Design review of the part built by this model. Coordinates are the model's own, in mm. Coordinates: 2 decimals unless noted, no trailing zeros. Write each loop counter-clockwise with the first axis right and the second up, starting at its lowest first coordinate (ties: lowest second). Pieces come first, ordered by that corner, then holes. Notation, with made-up numbers: M 86,12 L 120,12 A27 ccw 120,42 Z; hole C 40.5,28 d8. An arc over 180 degrees is marked long. One line per question, with ' | ' between items.
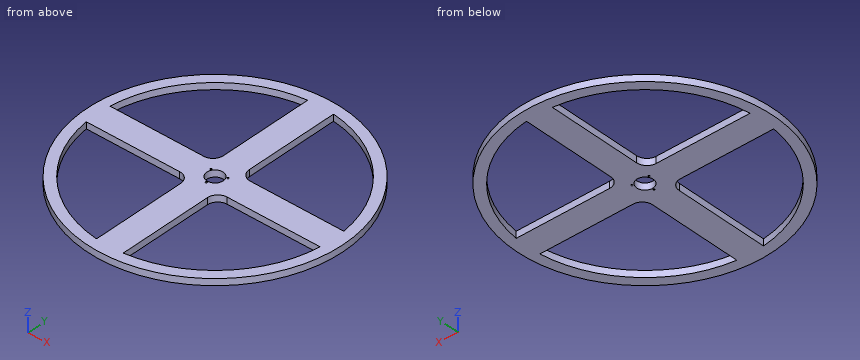
from build123d import *

# Parameters (mm, degrees)
SKETCH1_R           = 123.5325
SKETCH1_R_2         = 113.71
BOSS_EXTRUDE1_DEPTH = 6.35
CUT_EXTRUDE1_REACH  = 176.817
SKETCH2_R           = 7.937515
CUT_EXTRUDE2_REACH  = 176.817
SKETCH3_R           = 0.79375


with BuildPart() as part:
    # Sketch1 → Boss-Extrude1 (new body)
    # profile 1 of 2: a face of its own
    with BuildSketch(Plane.XY):
        Circle(SKETCH1_R)
        Circle(SKETCH1_R_2, mode=Mode.SUBTRACT)
    # profile 2 of 2: a face of its own
    with BuildSketch(Plane.XY):
        with BuildLine():
            ThreePointArc((22.7, 12.7), (15.628932188, 15.628932188), (12.7, 22.7))
            Line((12.7, 22.7), (12.7, 112.998557955))
            ThreePointArc((12.7, 112.998557955), (0.173278497, 113.709867974), (-12.355552704, 113.036739237))
            Line((-12.355552704, 113.036739237), (-12.355552704, 22.7))
            ThreePointArc((-12.355552704, 22.7), (-15.284484892, 15.628932188), (-22.355552704, 12.7))
            Line((-22.355552704, 12.7), (-112.998557955, 12.7))
            ThreePointArc((-112.998557955, 12.7), (-113.71, 0), (-112.998557955, -12.7))
            Line((-112.998557955, -12.7), (-22.7, -12.7))
            ThreePointArc((-22.7, -12.7), (-15.628932188, -15.628932188), (-12.7, -22.7))
            Line((-12.7, -22.7), (-12.7, -112.998557955))
            ThreePointArc((-12.7, -112.998557955), (0.173337872, -113.709867883), (13.044447296, -112.959313448))
            Line((13.044447296, -112.959313448), (13.044447296, -22.7))
            ThreePointArc((13.044447296, -22.7), (15.973379485, -15.628932188), (23.044447296, -12.7))
            Line((23.044447296, -12.7), (112.998557955, -12.7))
            ThreePointArc((112.998557955, -12.7), (113.53200017, -6.359955774), (113.71, 0))
            ThreePointArc((113.71, 0), (113.53200017, 6.359955774), (112.998557955, 12.7))
            Line((112.998557955, 12.7), (22.7, 12.7))
        make_face()
    extrude(amount=BOSS_EXTRUDE1_DEPTH)

    # Sketch2 → Cut-Extrude1 (cut, up to next)
    with BuildSketch(Plane.XY.offset(6.35), mode=Mode.PRIVATE) as cut_extrude1_sk1:
        Circle(SKETCH2_R)
    cut_extrude1_tool1 = extrude(cut_extrude1_sk1.sketch, amount=-CUT_EXTRUDE1_REACH, mode=Mode.PRIVATE) & part.part
    add(cut_extrude1_tool1.solids().sort_by_distance((0, 0, 6.35))[0], mode=Mode.SUBTRACT)

    # Sketch3 → Cut-Extrude2 (cut, up to next)
    with BuildSketch(Plane.XY.offset(6.35), mode=Mode.PRIVATE) as cut_extrude2_sk1:
        with Locations((0, -9.525)):
            Circle(SKETCH3_R)
    cut_extrude2_tool1 = extrude(cut_extrude2_sk1.sketch, amount=-CUT_EXTRUDE2_REACH, mode=Mode.PRIVATE) & part.part
    # Sketch3 → Cut-Extrude2 (cut, up to next)
    with BuildSketch(Plane.XY.offset(6.35), mode=Mode.PRIVATE) as cut_extrude2_sk2:
        with Locations((8.248891971, 4.7625)):
            Circle(SKETCH3_R)
    cut_extrude2_tool2 = extrude(cut_extrude2_sk2.sketch, amount=-CUT_EXTRUDE2_REACH, mode=Mode.PRIVATE) & part.part
    # Sketch3 → Cut-Extrude2 (cut, up to next)
    with BuildSketch(Plane.XY.offset(6.35), mode=Mode.PRIVATE) as cut_extrude2_sk3:
        with Locations((-8.248891971, 4.7625)):
            Circle(SKETCH3_R)
    cut_extrude2_tool3 = extrude(cut_extrude2_sk3.sketch, amount=-CUT_EXTRUDE2_REACH, mode=Mode.PRIVATE) & part.part
    add(cut_extrude2_tool1.solids().sort_by_distance((0, -9.525, 6.35))[0], mode=Mode.SUBTRACT)
    add(cut_extrude2_tool2.solids().sort_by_distance((8.248892, 4.7625, 6.35))[0], mode=Mode.SUBTRACT)
    add(cut_extrude2_tool3.solids().sort_by_distance((-8.248892, 4.7625, 6.35))[0], mode=Mode.SUBTRACT)


solid = part.part
1. To check wall thickness, follow line 1 along Y through (x, z) = (0, 1.75); line 2 along X through (y, z) = (50.5, 2); line 3 along X through (y, z) = (28, 4). State the ranges of each line that lie inside material, in increasing order. Write a range as [from, to].
Answer sheet:
line 1: [-123.53, -10.32], [-8.73, -7.94], [7.94, 123.53] | line 2: [-112.74, -101.88], [-12.36, 12.7], [101.88, 112.74] | line 3: [-120.32, -110.21], [-12.36, 12.7], [110.21, 120.32]
2. Take a section at B-B (x = 91.5). Write out the cut boundary in (y, z), then the cut area to 3 significant figures.
Answer sheet:
outline: M -82.99,0 L -67.51,0 L -67.51,6.35 L -82.99,6.35 Z; M -12.7,0 L 12.7,0 L 12.7,6.35 L -12.7,6.35 Z; M 67.51,0 L 82.99,0 L 82.99,6.35 L 67.51,6.35 Z | area: 358 mm^2
3. Take a section at A-A (y = 0). Write out the cut boundary in (x, z).
Answer sheet:
outline: M -123.53,0 L -7.94,0 L -7.94,6.35 L -123.53,6.35 Z; M 7.94,0 L 123.53,0 L 123.53,6.35 L 7.94,6.35 Z
4. Take a section at C-C (z = 3.25). Count the separate pieces of the cut face and the enclosed holes in it, then the cut area to 3 significant figures.
Answer sheet:
separate pieces: 1 | enclosed holes: 8 | area: 18,100 mm^2
5. Take a section at D-D (y = 102). Write out the cut boundary in (x, z).
Answer sheet:
outline: M -69.69,0 L -50.26,0 L -50.26,6.35 L -69.69,6.35 Z; M -12.36,0 L 12.7,0 L 12.7,6.35 L -12.36,6.35 Z; M 50.26,0 L 69.69,0 L 69.69,6.35 L 50.26,6.35 Z
6. Insertion check: pin 1 Ø3 at (y, z) = (-6, 1) entering from +X; pin 2 Ø3 at (y, z) = (74.5, 4.5) entering from +X; pin 3 Ø3 at (x, z) = (82.5, 4) entering from +Y. Each pin has a flat end and moves straight along its axis. Give the tip position at first contact, or say it passes through.
Answer sheet:
pin 1: x = 123.45 | pin 2: x = 99.66 | pin 3: y = 93.27
